Here's how the part is built. I have some questions about the finished solid (model axes, mm). A direction names the side the tool comes from. Round coordinates to 2 decimals unless told otherwise and drop trailing zeros. Loops run counter-clockwise (first coordinate to the right, second up) from the corner with the lowest first, then second, coordinate; pieces in that order, holes last. Notation, with made-up numbers: M 21,62 L 77,62 A17 cw 77,77 Z; hole C -30,32 d1. An arc over 180 degrees is marked long. Write item = value, one per line. Start each with the question number.
from build123d import *

# Parameters (mm, degrees)
F1_DEPTH = 6.35
F2_R     = 6.3499
F0_R     = 5.08
F3_DEPTH = 6.35


# Not quite as in the source:
# - a fillet or chamfer is up to 0.001 mm smaller than in the source, because OpenCascade refuses the exact size


with BuildPart() as f1:
    # F0 (on Front) → F1 (new body, symmetric)
    with BuildSketch(Plane.XZ):
        with BuildLine():
            Line((12.7, 6.35), (-12.7, 6.35))
            Line((-12.7, 6.35), (-12.7, -6.35))
            Line((-12.7, -6.35), (12.7, -6.35))
            ThreePointArc((12.7, -6.35), (10.471147458, 0), (12.7, 6.35))
        make_face()
        with BuildLine():
            Line((-12.7, -6.35), (-12.7, 6.35))
            ThreePointArc((-12.7, 6.35), (-19.05, 0), (-12.7, -6.35))
        make_face()
    extrude(amount=F1_DEPTH, both=True)

    # F2 (radius 6.35 in the source; OpenCascade refuses exactly that, so slightly less here)
    f2_edges = [f1.edges().sort_by_distance(p)[0] for p in [
        (0, -6.35, 6.35),
        (0, 6.35, 6.35),
        (0, -6.35, -6.35),
        (0, 6.35, -6.35),
    ]]
    fillet(f2_edges, radius=F2_R)

    # F0 (on Front) → F3 (join)
    with BuildSketch(Plane.XZ):
        with BuildLine():
            ThreePointArc((30.791147458, 0), (23.9960502669, 9.5866067556), (12.7, 6.35))
            Line((12.7, 6.35), (12.7, -6.35))
            ThreePointArc((12.7, -6.35), (23.9960502669, -9.5866067556), (30.791147458, 0))
        make_face()
        with Locations((20.631147458, 0)):
            Circle(F0_R, mode=Mode.SUBTRACT)
        with BuildLine():
            Line((12.7, -6.35), (12.7, 6.35))
            ThreePointArc((12.7, 6.35), (10.471147458, 0), (12.7, -6.35))
        make_face()
    extrude(amount=F3_DEPTH)


solid = f1.part
Item 1: Please list where these lines run through material, in increasing order: line 1 (Y direction, x = 17.5, z = 7.75); line 2 (X direction, y = -3.5, z = -0.75); line 3 (X direction, y = -2, z = 1). Write a range as [from, to].
Item 2: I want a section at C-C, the plane z = 8. List the corners of the cut face in (x, y) for me.
Item 3: Will these pins go through, and if not, where does the flat tip stop? pin 1 Ø4 at (x, y) = (9, -3.5) entering from +Z; pin 2 Ø1 at (x, y) = (5, -4.5) entering from +Z; pin 3 Ø3 at (y, z) = (2, -3) entering from +X; pin 4 Ø9 at (x, z) = (20.63, 0) entering from -Y.
Item 4: For faces 4 (the cylindrical face through (-0.18, -4.44, 4.54)), 5 (the cylindrical face through (0.18, -4.44, -4.54)), 6 (the cylindrical face through (0.18, 4.44, -4.54)), which set-ups out of +Z, -Z, +X, -X, +Y, -Y let a thin tool reach every point of the face, with its end or its side?
Item 5: I want a section at A-A, the plane x = 18.5. List the corners of the cut face in (y, z) for me.
Item 6: I want a section at B-B, the plane x = 24. List the corners of the cut face in (y, z) for me.
Item 7: We'd pull the mould along X, two halves only. Please class faces 1 (the flat face through (23, 0, 5)), 2 (the cylindrical face through (25.477, -3.131, 1.526)), 3 (the cylindrical face through (10.47, 2.42, -0.1)): released by +X, released by -X, zero draft, split by the parting line, or undercut.
Worked out:
q1.line_1 = [-6.35, 0]
q1.line_2 = [-17.95, 15.61], [25.66, 30.76]
q1.line_3 = [-18.64, 15.65], [25.61, 30.74]
q2.outline = M 14.37,-6.35 L 26.89,-6.35 L 26.89,0 L 14.37,0 Z
q3.pin_1 = 6.17
q3.pin_2 = 4.93
q3.pin_3 = 11.52
q3.pin_4 = through
q4.face_4 = +Z, -X, -Y
q4.face_5 = -Z, -X, -Y
q4.face_6 = -Z, +X, -X, +Y
q5.outline = M -6.35,-9.93 L 0,-9.93 L 0,-4.61 L -6.35,-4.61 Z; M -6.35,4.61 L 0,4.61 L 0,9.93 L -6.35,9.93 Z
q6.outline = M -6.35,-9.59 L 0,-9.59 L 0,-3.8 L -6.35,-3.8 Z; M -6.35,3.8 L 0,3.8 L 0,9.59 L -6.35,9.59 Z
q7.face_1 = zero draft
q7.face_2 = undercut
q7.face_3 = released by +X
